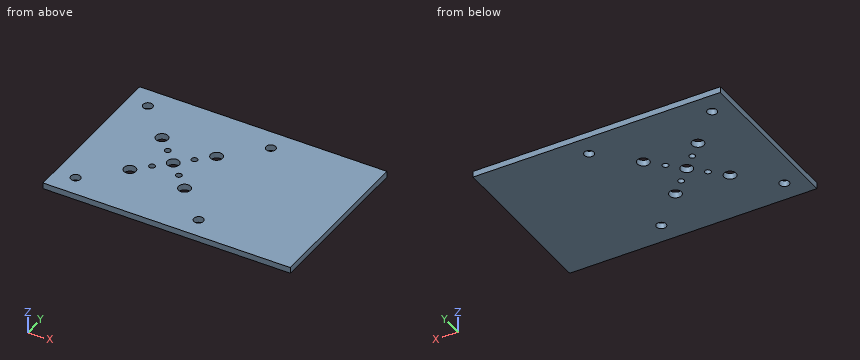
Solid Edge part; units mm, degrees
sketch "Sketch1" plane through (0, 0, 0) normal (0, 0, 1) x (1, 0, 0)
  line L0 (40, -25) -> (40, 30)
  line L1 (40, 30) -> (-42.5, 30)
  line L2 (-42.5, 30) -> (-42.5, -25)
  line L3 (-42.5, -25) -> (40, -25)
extrude "ExtrudedProtrusion_3" add sketch "Sketch1" along normal blind 2
sketch "Sketch2" plane through (0, 0, 0) normal (0, 0, 1) x (1, 0, 0)
  circle A0 centre (-35.6965, 23.0215) radius 1.6
  circle A1 centre (5.3589, 23.016) radius 1.6
  circle A2 centre (5.346, -18.0319) radius 1.6
  circle A3 centre (-35.7266, -17.9943) radius 1.6
  circle A4 centre (-24.2914, -6.6214) radius 2
  circle A5 centre (-19.6326, -1.9626) radius 1
  circle A6 centre (-6.0516, -6.6214) radius 2
  circle A7 centre (-10.7104, -1.9626) radius 1
  circle A8 centre (-15.1715, 2.4985) radius 2
  circle A9 centre (-10.7104, 6.9596) radius 1
  circle A10 centre (-6.0516, 11.6184) radius 2
  circle A11 centre (-19.6326, 6.9596) radius 1
  circle A12 centre (-24.2914, 11.6184) radius 2
extrude "ExtrudedCutout_14" cut sketch "Sketch2" along normal blind 2
properties material "ABS Plastic, high impact"
Geometry check sheet. Reference: the model listing, model coordinates, mm. Coordinates: 2 decimals unless noted, no trailing zeros. Write each loop counter-clockwise with the first axis right and the second up, starting at its lowest first coordinate (ties: lowest second). Pieces come first, ordered by that corner, then holes. Notation, with made-up numbers: M 55,36 L 99,36 A32 cw 99,74 Z; hole C 89.25,-34 d3. An arc over 180 degrees is marked long. Answer as a JSON object with one key per item and string values.
1. Section check A-A, the plane x = -25. Enter the section's corners in (y, z), plus the area to 3 significant figures.
Answers below:
{"outline": "M -25,0 L -8.49,0 L -8.49,2 L -25,2 Z; M -4.75,0 L 9.75,0 L 9.75,2 L -4.75,2 Z; M 13.49,0 L 30,0 L 30,2 L 13.49,2 Z", "area": "95.0 mm²"}
2. Scan lines: L1, parallel to Y at x = 5.5, z = 0.3; L2, parallel to X at y = 22, z = 1.2; L3, parallel to X at y = -7.5, z = 0.75. Record each from-to range of solid material in increasing order.
Answers below:
{"L1": "y = -25 to -19.62, -16.44 to 21.42, 24.61 to 30", "L2": "x = -42.5 to -36.93, -34.47 to 4.12, 6.59 to 40", "L3": "x = -42.5 to -26.09, -22.49 to -7.85, -4.25 to 40"}
3. Go/stop test with a flat-tipped pin: pin 1 Ø1.2 at (x, y) = (-10.71, 6.96) entering from +Z. Record where the tip stops, or that it passes through.
Answers below:
{"pin 1": "passes through"}
4. Section check B-B, the plane z = 1.05. Give the number of separate pieces and of enclosed holes in the cut face, plus the area to 3 significant figures.
Answers below:
{"separate pieces": "1", "enclosed holes": "13", "area": "4,430 mm²"}
5. Section check C-C, the plane x = -6. Enter the section's corners in (y, z), plus the area to 3 significant figures.
Answers below:
{"outline": "M -25,0 L -8.62,0 L -8.62,2 L -25,2 Z; M -4.62,0 L 9.62,0 L 9.62,2 L -4.62,2 Z; M 13.62,0 L 30,0 L 30,2 L 13.62,2 Z", "area": "94.0 mm²"}
